Can you work these out from the drawing? Everything is in mm from the part's minimum corner. Give positions to 0.01 mm unless a question says otherwise; leave off trailing zeros. Loops run counter-clockwise (first coordinate to the right, second up) from the corner with the lowest first, then second, coordinate; pieces in that order, holes last.
Q1. If we section it at B-B (y = 30): Please give me the cut outline in (x, z), plus the area to 3 significant figures.
Q2. If we section it at D-D (x = 29): Please give me the cut outline in (y, z).
Q3. Will these pins go through, and if not, where does the flat tip stop? P1, Ø12, axis at x = 14, y = 30.5, coming from the +Z side; P2, Ø0.9, axis at y = 28.5, z = 2, coming from the -X side; P3, Ø1, axis at x = 23.5, z = 1.5, coming from the +Y side.
Q4. I need wall thicknesses on line 1 (X direction, y = 30, z = 2.15); line 2 (Y direction, x = 65, z = 1.6); line 3 (X direction, y = 10, z = 2). Which ranges of each line are inside material? Lowest first, please.
Q5. If we section it at A-A (x = 65): Please give me the cut outline in (y, z), plus the area to 3 significant figures.
Q6. If we section it at C-C (z = 0.5): Please give me the cut outline in (x, y).
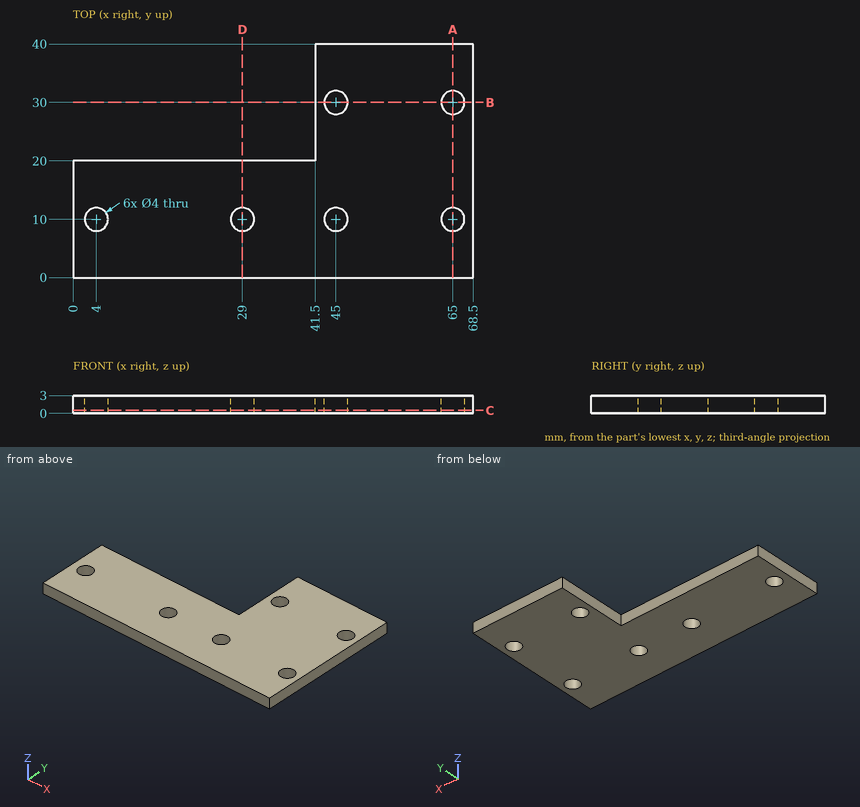
Check sheet entries:
1. outline: (41.5, 0) - (43, 0) - (43, 3) - (41.5, 3) - close; (47, 0) - (63, 0) - (63, 3) - (47, 3) - close; (67, 0) - (68.5, 0) - (68.5, 3) - (67, 3) - close
1. area: 57.0 mm2
2. outline: (0, 0) - (8, 0) - (8, 3) - (0, 3) - close; (12, 0) - (20, 0) - (20, 3) - (12, 3) - close
3. P1: passes through
3. P2: stops at x = 41.5
3. P3: stops at y = 20
4. line 1: x = 41.5 to 43, 47 to 63, 67 to 68.5
4. line 2: y = 0 to 8, 12 to 28, 32 to 40
4. line 3: x = 0 to 2, 6 to 27, 31 to 43, 47 to 63, 67 to 68.5
5. outline: (0, 0) - (8, 0) - (8, 3) - (0, 3) - close; (12, 0) - (28, 0) - (28, 3) - (12, 3) - close; (32, 0) - (40, 0) - (40, 3) - (32, 3) - close
5. area: 96.0 mm2
6. outline: (0, 0) - (68.5, 0) - (68.5, 40) - (41.5, 40) - (41.5, 20) - (0, 20) - close; hole circle Ø4 at (4, 10); hole circle Ø4 at (29, 10); hole circle Ø4 at (45, 10); hole circle Ø4 at (45, 30); hole circle Ø4 at (65, 10); hole circle Ø4 at (65, 30)
